from build123d import *

# Parameters (mm, degrees)
SKETCH1_W           = 18
SKETCH1_H           = 13
BOSS_EXTRUDE1_DEPTH = 1.5
SKETCH2_R           = 0.5
BOSS_EXTRUDE2_DEPTH = 5
CUT_EXTRUDE1_REACH  = 3.5
SKETCH3_R           = 1.5


with BuildPart() as part:
    # Sketch1 → Boss-Extrude1 (new body)
    with BuildSketch(Plane.XY):
        with Locations((165.583059714, 53.307197022)):
            Rectangle(SKETCH1_W, SKETCH1_H)
    extrude(amount=BOSS_EXTRUDE1_DEPTH)

    # Sketch2 → Boss-Extrude2 (add)
    with BuildSketch(Plane.XY.offset(1.5)):
        with Locations((158.334176002, 53.307197022)):
            Circle(SKETCH2_R)
        with Locations((158.334176002, 55.307197022)):
            Circle(SKETCH2_R)
        with Locations((158.334176002, 57.307197022)):
            Circle(SKETCH2_R)
        with Locations((158.334176002, 51.307197022)):
            Circle(SKETCH2_R)
        with Locations((158.334176002, 49.307197022)):
            Circle(SKETCH2_R)
    extrude(amount=BOSS_EXTRUDE2_DEPTH)

    # Sketch3 → Cut-Extrude1 (cut, up to next)
    with BuildSketch(Plane.XY.offset(1.5), mode=Mode.PRIVATE) as cut_extrude1_sk1:
        with Locations((172.583059714, 57.557197022)):
            Circle(SKETCH3_R)
    cut_extrude1_tool1 = extrude(cut_extrude1_sk1.sketch, amount=-CUT_EXTRUDE1_REACH, mode=Mode.PRIVATE) & part.part
    add(cut_extrude1_tool1.solids().sort_by_distance((172.58306, 57.557197, 1.5))[0], mode=Mode.SUBTRACT)
    # Sketch3 → Cut-Extrude1 (cut, up to next)
    with BuildSketch(Plane.XY.offset(1.5), mode=Mode.PRIVATE) as cut_extrude1_sk2:
        with Locations((172.583059714, 49.057197022)):
            Circle(SKETCH3_R)
    cut_extrude1_tool2 = extrude(cut_extrude1_sk2.sketch, amount=-CUT_EXTRUDE1_REACH, mode=Mode.PRIVATE) & part.part
    add(cut_extrude1_tool2.solids().sort_by_distance((172.58306, 49.057197, 1.5))[0], mode=Mode.SUBTRACT)


solid = part.part
Verification items for the finished model (mm, model axes). A direction names the side the tool comes from. Coordinates: 2 decimals unless noted, no trailing zeros. Write each loop counter-clockwise with the first axis right and the second up, starting at its lowest first coordinate (ties: lowest second). Pieces come first, ordered by that corner, then holes. Notation, with made-up numbers: (-23.75, -39) -> (28.25, -39) arc R28 cw to (28.25, -2) -> close; hole circle Ø11 at (-20.75, -12). An arc over 180 degrees is marked (long way). One line per item, written item: value. Start each with the question number.
Q1. Mould release check, pull along X, two halves, no side actions. Record for faces 1 (the cylindrical face through (172.388, 59.044, 0.76)), 2 (the cylindrical face through (157.835, 55.329, 3.965)), 3 (the flat face through (165, 53, 0)): pulls with the +X half, pulls with the -X half, needs draft (parallel to the pull), parting line crosses it, or undercut.
Q2. Cross-section at A-A on y = 50.25. Enter the section's corners in (x, z).
Q3. Access from +Z, -Z, +X, -X, +Y, -Y to the whole of each face (thin tool, end or side, straight path). Record for faces 4 (the cylindrical face through (157.835, 53.329, 3.965)), 5 (the flat face through (158.3, 55.3, 6.5)).
Q4. Go/stop test with a flat-tipped pin: P1, Ø4, axis at x = 172.58, y = 57.56, coming from the +Z side. Record where the tip stops, or that it passes through.
Q5. Cross-section at B-B on x = 172.25. Enter the section's corners in (y, z).
Q6. Cross-section at D-D on y = 58. Enter the section's corners in (x, z).
Q7. Cross-section at C-C on z = 4.25. Enter the section's corners in (x, y), and give its area (3 significant figures).
Q8. Thickness scan on L1, parallel to Z at x = 158, y = 48.5; L2, parallel to X at y = 58, z = 1.25; L3, parallel to X at y = 53, z = 6.25. Record the ranges inside material, lowest first. Write a range as from..to.
Checked values:
1. face 1: undercut
1. face 2: parting line crosses it
1. face 3: needs draft
2. outline: (156.58, 0) -> (171.67, 0) -> (171.67, 1.5) -> (156.58, 1.5) -> close; (173.49, 0) -> (174.58, 0) -> (174.58, 1.5) -> (173.49, 1.5) -> close
3. face 4: +Z
3. face 5: +Z, +X, -X, +Y, -Y
4. P1: stops at z = 1.5
5. outline: (46.81, 0) -> (47.59, 0) -> (47.59, 1.5) -> (46.81, 1.5) -> close; (50.52, 0) -> (56.09, 0) -> (56.09, 1.5) -> (50.52, 1.5) -> close; (59.02, 0) -> (59.81, 0) -> (59.81, 1.5) -> (59.02, 1.5) -> close
6. outline: (156.58, 0) -> (171.15, 0) -> (171.15, 1.5) -> (156.58, 1.5) -> close; (174.02, 0) -> (174.58, 0) -> (174.58, 1.5) -> (174.02, 1.5) -> close
7. outline: circle Ø1 at (158.33, 49.31); circle Ø1 at (158.33, 51.31); circle Ø1 at (158.33, 53.31); circle Ø1 at (158.33, 55.31); circle Ø1 at (158.33, 57.31)
7. area: 3.93 mm²
8. L1: z = 0..1.5
8. L2: x = 156.58..171.15, 174.02..174.58
8. L3: x = 157.94..158.73
